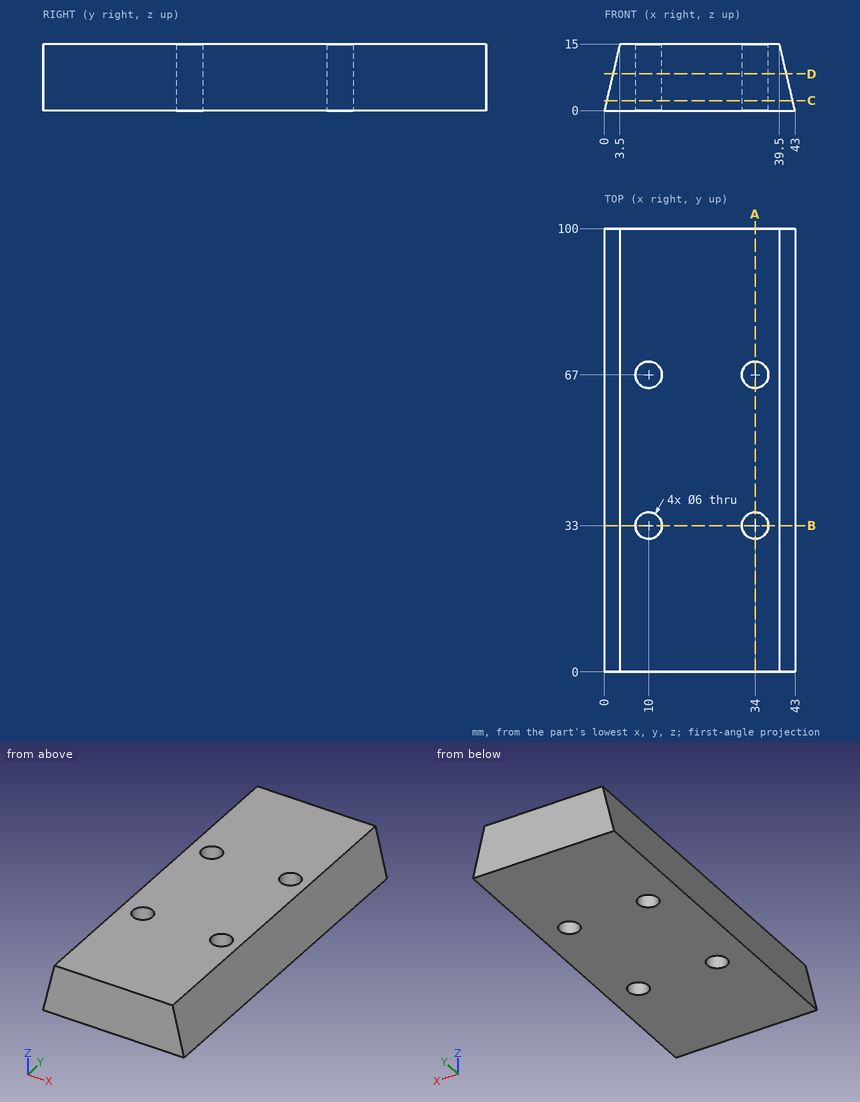
Design review of the part shown in the three views and the two pictorial views. Dimensions are in mm from the part's minimum x, y and z. Give positions to 0.01 mm unless a question says otherwise; leave off trailing zeros. Write each loop counter-clockwise with the first axis right and the second up, starting at its lowest first coordinate (ties: lowest second). Pieces come first, ordered by that corner, then holes. Notation, with made-up numbers: M -37.75,-4.75 L -11.75,-4.75 A27 ccw -11.75,16.25 Z; hole C 13,40.25 d5. An arc over 180 degrees is marked long. Answer in a Markdown table with one row per item.
Item 1: Add section B-B on y = 33. Give the boundary of the cut face in (x, z), plus the area to 4 significant figures.
Check sheet entries:
| item | result |
|---|---|
| outline | M 0,0 L 7,0 L 7,15 L 3.5,15 Z; M 13,0 L 31,0 L 31,15 L 13,15 Z; M 37,0 L 43,0 L 39.5,15 L 37,15 Z |
| area | 412.5 mm2 |
Item 2: For P1, Ø1.5, axis at y = 85, z = 2.5, coming from the -X side; P2, Ø5.5, axis at x = 34, y = 67, coming from the +Z side, all flat-tipped, find the tip position at first contact; note any pin that passes through.
Check sheet entries:
| item | result |
|---|---|
| P1 | x = 0.41 |
| P2 | through |
Item 3: Add section C-C on z = 2.25. Give the boundary of the cut face in (x, y) (3 decimals).
Check sheet entries:
| item | result |
|---|---|
| outline | M 0.525,0 L 42.475,0 L 42.475,100 L 0.525,100 Z; hole C 10,33 d6; hole C 10,67 d6; hole C 34,33 d6; hole C 34,67 d6 |
Item 4: Add section A-A on x = 34. Give the boundary of the cut face in (y, z), plus the area to 3 significant figures.
Check sheet entries:
| item | result |
|---|---|
| outline | M 0,0 L 30,0 L 30,15 L 0,15 Z; M 36,0 L 64,0 L 64,15 L 36,15 Z; M 70,0 L 100,0 L 100,15 L 70,15 Z |
| area | 1,320 mm2 |
Item 5: For line 1 along Y through (x, z) = (10, 4); line 2 along Y through (x, z) = (8.5, 12.5); line 3 along X through (y, z) = (67, 10), list the stretches that pass through material, from the lowest coordinate up.
Check sheet entries:
| item | result |
|---|---|
| line 1 | 0 to 30, 36 to 64, 70 to 100 |
| line 2 | 0 to 30.4, 35.6 to 64.4, 69.6 to 100 |
| line 3 | 2.33 to 7, 13 to 31, 37 to 40.67 |
Item 6: Add section D-D on z = 8.25. Give the boundary of the cut face in (x, y) (3 decimals), plus the area to 3 significant figures.
Check sheet entries:
| item | result |
|---|---|
| outline | M 1.925,0 L 41.075,0 L 41.075,100 L 1.925,100 Z; hole C 10,33 d6; hole C 10,67 d6; hole C 34,33 d6; hole C 34,67 d6 |
| area | 3,800 mm2 |
